For this review, take the finished solid that the model builds, in its own axes (mm). Face numbers are marked on the shaded views. A direction names the side the tool comes from. Coordinates: 2 decimals unless noted, no trailing zeros. Loops run counter-clockwise (first coordinate to the right, second up) from the corner with the lowest first, then second, coordinate; pieces in that order, holes last. Notation, with made-up numbers: (46.5, -21) - (64.5, -21) arc R28 cw to (64.5, -3) - close; hole circle Ø2 at (56.25, -36). An arc over 180 degrees is marked (long way). One line per item, written item: value. Start each with the question number.
1. Insertion check: pin 1 (0.7 mm diameter, centred on x = -1, z = 0, fed in from +Y); pin 2 (2 mm diameter, centred on y = -0.5, z = -2, fed in from +X). Each pin has a flat end and moves straight along its axis. Give the tip position at first contact, or say it passes through.
2. For the marked faces 4 and 5, list the 3-axis set-ups (+Z, -Z, +X, -X, +Y, -Y) from which the entire face can be reached by the end or side of a thin tool; tool diameter is ignored.
3. The part is to be moulded in two halves that separate along Y. For the marked faces 1, 2 and 3, say which applies: released by +Y, released by -Y, zero draft, split by the parting line, or undercut.
4. Take a section at A-A, the plane x = 2.5. State the section outline as (y, z) points, and give its area (3 significant figures).
5. To check wall thickness, follow line 1 (Y direction, x = -1, z = 0.7); line 2 (Z direction, x = -1, y = 0.45); line 3 (Y direction, x = -0.75, z = -0.3). State the ranges of each line that lie inside material, in increasing order. Write a range as from..to.
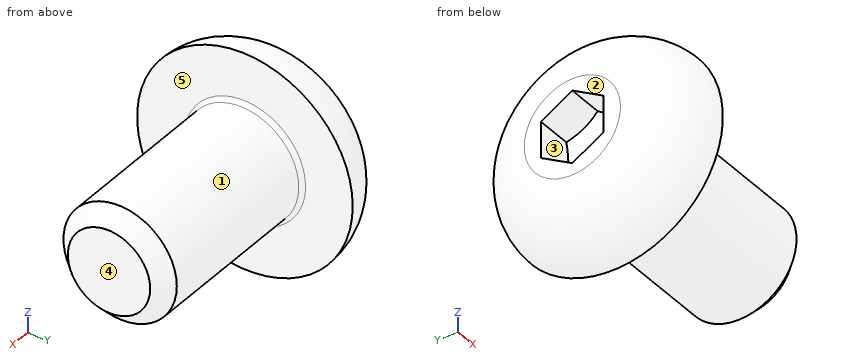
Autodesk Inventor part; units mm, degrees
ref_plane "Work Plane1" through (29, 0, 0) normal (0, -1, 0) x (1, 0, 0)
ref_plane "YZ Plane" through (0, 0, 0) normal (1, 0, 0) x (0, 1, 0)
ref_plane "XZ Plane" through (0, 0, 0) normal (0, 1, 0) x (-1, 0, 0)
sketch "Sketch1" plane through (0, 0, 0) normal (0, 0, 1) x (1, 0, 0)
  line L0 (-0.0847, 0) -> (4.7625, 0)
  line L1 (4.7625, 0) -> (4.7625, 1.4224)
  line L2 (4.7625, 1.4224) -> (1.2702, 1.4224)
  line L3 (1.2702, 1.4224) -> (0.0001, 1.4224)
  line L4 (0.0001, 1.4224) -> (0, 1.4224)
  line L5 (0, 1.4224) -> (0, 2.7051)
  line L6 (0, 2.7051) -> (-1.4986, 2.7051)
  line L7 (-1.4986, 2.7051) -> (-1.4986, 0.9092)
  line L8 (-1.4986, 0.9092) -> (-0.6096, 0.9092)
  line L9 (-0.6096, 0.9092) -> (-0.0847, 0)
  line L10 (-2.7508, 0) -> (6.0147, 0)
  line L11 (0, -0.541) -> (0, 3.2461)
  line L12 (1.2702, 1.4224) -> (0, 1.4224) construction
  dimension "d1" = 3.4923
  dimension "d2" = 1.2701
  dimension "d3" = 1.4986
  dimension "d4" = 0.889
  dimension "d5" = 60
  dimension "d6" = 2.8448
  dimension "d7" = 2.8448
  dimension "d8" = 1.8184
  dimension "d9" = 5.4102
  dimension "d26" = 4.7625
revolve "Body" add sketch "Sketch1" angle 360 about axis through (-0.0847, 0, 0) along (1, 0, 0)
sketch "Sketch2" plane through (-1.4986, 0, 0) normal (-1, 0, 0) x (0, 0, 1)
  circle A0 centre (0, 0) radius 0.9092
  line L0 (0, -3.7871) -> (0, 3.7871)
  line L1 (-3.7871, 0) -> (3.7871, 0)
  line L2 (0.9092, 0) -> (0.4546, -0.7874)
  line L3 (0.4546, -0.7874) -> (-0.4546, -0.7874)
  line L4 (-0.4546, -0.7874) -> (-0.9092, 0)
  line L5 (-0.9092, 0) -> (-0.4546, 0.7874)
  line L6 (-0.4546, 0.7874) -> (0.4546, 0.7874)
  line L7 (0.4546, 0.7874) -> (0.9092, 0)
extrude "Slot" add sketch "Sketch2" against normal up to next contours L7 A0 | A0 L2 | L6 L0 A0 | A0 L0 L3 | L0 L6 A0 | A0 L3 L0 | L4 A0 | A0 L5
fillet "Fillet1" radius 1.4985 1 edges at (-1.4986, -2.7051, 0)
thread "Thread"
chamfer "Chamfer1" distance 0.3895 distance2 0.3896 1 edges at (4.7625, -1.4224, 0) measured on face at (4.7625, -0.0627, 0.6443)
ref_plane "Work Plane1" through (29, 0, 0) normal (0, -1, 0) x (1, 0, 0)
fillet "Fillet2" radius 0.1 1 edges at (0.0001, -1.4224, 0)
equation "\"d1\" = GEL"
equation "\"d3\" = KOH"
equation "\"d4\" = INTI"
equation "\"d6\" = GD"
equation "\"d7\" = BDM"
equation "\"d8\" = 1.1547 * SW"
equation "\"d9\" = KOD"
equation "\"d26\" = NLG"
equation "\"d30\" = R"
equation "\"d17\" = RR"
equation "\"d13\" = GEL"
equation "\"d15\" = -0.5 * SPD + 0.5 * GD"
equation "\"d16\" = GUL"
equation "\"GD\" = NND"
equation "\"NLG\" = 4.7625"
equation "\"GEL\" = 3.4923"
equation "\"KOD\" = 5.4102"
equation "\"KOH\" = 1.4986"
equation "\"INTI\" = 0.889"
equation "\"GAL\" = 1.27"
equation "\"GUL\" = 0.38964"
equation "\"BDM\" = NND"
equation "\"SW\" = 1.5748"
equation "\"RR\" = 1.4985"
equation "\"SPD\" = 2.06578"
equation "\"R\" = 0.1"
equation "\"TOA\" = 30deg"
equation "\"GD1\" = SPD"
equation "\"THREADDIA\" = 2.8448"
equation "\"KOH1\" = 0.381"
equation "\"NND\" = 2.8448"
equation "\"E0\" = 1.81889"
properties part number "ANSI B18.3 - 4 - 40 x 3/16, HSBHCSI" material "Steel, Mild"
Solutions:
1. pin 1: y = 2.56
1. pin 2: x = 4.73
2. face 4: +Z, -Z, +X, +Y, -Y
2. face 5: +X
3. face 1: split by the parting line
3. face 2: zero draft
3. face 3: undercut
4. outline: circle Ø2.84 at (0, 0)
4. area: 6.36 mm2
5. line 1: -2.21..-0.36, 0.36..2.21
5. line 2: -2.28..-0.65, 0.65..2.28
5. line 3: -2.49..-0.79, 0.79..2.49
